```python
from build123d import *

# Parameters (mm, degrees)
SKETCH1_R           = 31.5
BOSS_EXTRUDE1_DEPTH = 11
SKETCH2_R           = 3.25
CUT_EXTRUDE1_DEPTH  = 46.885727629
SKETCH3_R           = 6
CUT_EXTRUDE2_DEPTH  = 5
CHAMFER1_SIZE       = 0.5
SKETCH4_R           = 15.75
BOSS_EXTRUDE2_DEPTH = 2
CHAMFER2_SIZE       = 0.5
CIRPATTERN1_COUNT   = 4
M5_TAPPED_HOLE1_D   = 4.2


with BuildPart() as part:
    # Sketch1 → Boss-Extrude1 (new body)
    with BuildSketch(Plane(origin=(0, 0, 0), x_dir=(0, 0, -1), z_dir=(1, 0, 0))):
        Circle(SKETCH1_R)
    extrude(amount=BOSS_EXTRUDE1_DEPTH)

    # Sketch2 → Cut-Extrude1 (cut, through all)
    with BuildSketch(Plane.ZY):
        with Locations((0, 25)):
            Circle(SKETCH2_R)
        with Locations((0, -25)):
            Circle(SKETCH2_R)
    cut_extrude1 = extrude(amount=-CUT_EXTRUDE1_DEPTH, mode=Mode.SUBTRACT)

    # Sketch3 → Cut-Extrude2 (cut)
    with BuildSketch(Plane.ZY):
        with Locations((0, 25)):
            Circle(SKETCH3_R)
        with Locations((0, -25)):
            Circle(SKETCH3_R)
    cut_extrude2 = extrude(amount=-CUT_EXTRUDE2_DEPTH, mode=Mode.SUBTRACT)

    # Chamfer1
    chamfer1_edges = [part.edges().sort_by_distance(p)[0] for p in [
        (0, 0, 31.5),
        (11, 0, 31.5),
    ]]
    chamfer(chamfer1_edges, length=CHAMFER1_SIZE - 0.0001)  # a hair under: the kernel refuses the full size

    # Sketch4 → Boss-Extrude2 (add)
    with BuildSketch(Plane(origin=(11, 0, 0), x_dir=(0, 0, -1), z_dir=(1, 0, 0))):
        Circle(SKETCH4_R)
    extrude(amount=BOSS_EXTRUDE2_DEPTH)

    # Chamfer2
    chamfer2_edges = [part.edges().sort_by_distance(p)[0] for p in [
        (13, 0, 15.75),
    ]]
    chamfer(chamfer2_edges, length=CHAMFER2_SIZE)

    # CirPattern1: Cut-Extrude1, Cut-Extrude2 ×4 about axis
    cirpattern1_axis = Axis((0, 0, 0), (1, 0, 0))
    add([cut_extrude1.rotate(cirpattern1_axis, i * 360 / CIRPATTERN1_COUNT) for i in range(1, CIRPATTERN1_COUNT)], mode=Mode.SUBTRACT)
    add([cut_extrude2.rotate(cirpattern1_axis, i * 360 / CIRPATTERN1_COUNT) for i in range(1, CIRPATTERN1_COUNT)], mode=Mode.SUBTRACT)

    # M5 Tapped Hole1 (through all)
    with Locations(Plane(origin=(0, 17.67766953, -17.67766953), x_dir=(0, 0, -1), z_dir=(-1, 0, 0))):
        with Locations((0, 0), (-35.35533906, 0), (0, 35.35533906), (-35.35533906, 35.35533906)):
            Hole(M5_TAPPED_HOLE1_D / 2)


solid = part.part
```
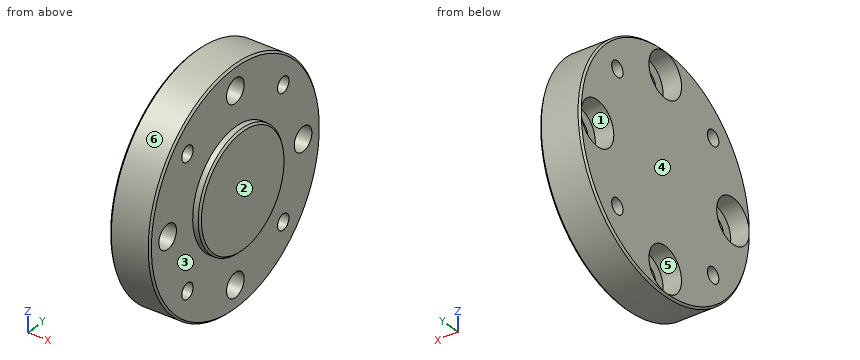
Read the model definition and answer for the solid it produces. Units are mm, in the model's axes. Face numbers are marked on the shaded views. A direction names the side the tool comes from. Give positions to 0.01 mm unless a question says otherwise; leave off trailing zeros.
Item 1: Each of these flat-tipped pins is pushed along its axis until it touches: pin 1 Ø1.5 at (x, y) = (5.5, 24) entering from +Z; pin 2 Ø3.5 at (y, z) = (-24, -2) entering from -X; pin 3 Ø4 at (x, z) = (3, -21) entering from -Y. Where does it stop, or does it pass through?
Item 2: The part is cut by section A-A (y = 0). Give the number of separate pieces and of enclosed holes in the cut face, and give its area (3 significant figures).
Item 3: Find the intervals of material crossed by line 1 along Y through (x, z) = (3.65, 0); line 2 along Y through (x, z) = (6.3, 0); line 3 along Y through (x, z) = (4.25, -19.5), in increasing order.
Item 4: The mould has two halves that part along Z. Classify the marked faces 4, 5 and 6: released by +Z, released by -Z, zero draft, split by the parting line, or undercut.
Item 5: For the marked faces 1, 2 and 3, determine the directions among +Z, -Z, +X, -X, +Y, -Y from which every point of the face is accessible in a straight line to the end or side of a thin tool.
Taken from the geometry:
1. pin 1: stops at z = 21.25
1. pin 2: stops at x = 5
1. pin 3: stops at y = -25.12
2. separate pieces: 3
2. enclosed holes: 0
2. area: 557 mm2
3. line 1: y = -31.5 to -31, -19 to 19, 31 to 31.5
3. line 2: y = -31.5 to -28.25, -21.75 to 21.75, 28.25 to 31.5
3. line 3: y = -24.74 to -18.72, -16.63 to -2.4, 2.4 to 16.63, 18.72 to 24.74
4. face 4: zero draft
4. face 5: undercut
4. face 6: split by the parting line
5. face 1: -X
5. face 2: +Z, -Z, +X, +Y, -Y
5. face 3: +X
